from build123d import *


with BuildPart() as f1:
    # F0 (on Front) → F1 (revolve)
    with BuildSketch(Plane.XZ):
        with BuildLine():
            ThreePointArc((9, 2), (9.736068, 1.118034), (10, 0))
            Line((10, 0), (11, 0))
            Line((11, 0), (11, 3.25))
            ThreePointArc((11, 3.25), (10.926777, 3.426777), (10.75, 3.5))
            Line((10.75, 3.5), (9.606548, 3.5))
            ThreePointArc((9.606548, 3.5), (9.429771, 3.426777), (9.356548, 3.25))
            Line((9.356548, 3.25), (9.356548, 3))
            Line((9.356548, 3), (9, 3))
            Line((9, 3), (9, 2))
        make_face()
        with BuildLine():
            Line((11, 0), (10, 0))
            ThreePointArc((10, 0), (9.736068, -1.118034), (9, -2))
            Line((9, -2), (9, -3))
            Line((9, -3), (9.356548, -3))
            Line((9.356548, -3), (9.356548, -3.25))
            ThreePointArc((9.356548, -3.25), (9.429771, -3.426777), (9.606548, -3.5))
            Line((9.606548, -3.5), (10.75, -3.5))
            ThreePointArc((10.75, -3.5), (10.926777, -3.426777), (11, -3.25))
            Line((11, -3.25), (11, 0))
        make_face()
    revolve(axis=Axis((0, 0, -0.050428), (0, 0, -1)))


solid = f1.part
Part model, mm, in its own coordinate system. Coordinates: 2 decimals unless noted, no trailing zeros. Loops run counter-clockwise (first coordinate to the right, second up) from the corner with the lowest first, then second, coordinate; pieces in that order, holes last. Notation, with made-up numbers: (-21.75, -10) -> (-6.75, -10) arc R19 cw to (-6.75, 14) -> close; hole circle Ø9 at (65, 45). An arc over 180 degrees is marked (long way). Use a Markdown table: item, result. Add a question column.
Item 1: Pull direction Y, two halves, no side cores. Call faces 1 (the cylindrical face through (-1.172, -8.923, -2.507)), 2 (the cylindrical face through (-1.172, -8.923, 2.493)), 3 (the flat face through (-8, 6, 3.5)), 4 (the cylindrical face through (-2.38, 10.74, 0.05)): +Y half, -Y half, draft (parallel to the pull), parting line (faces both ways), or undercut.
Item 2: Flat gauge pins, fed straight in: P1, Ø4, axis at y = -3.5, z = -2.5, coming from the -X side; P2, Ø1, axis at y = -7.5, z = -0.5, coming from the -X side; P3, Ø2, axis at x = -6.5, z = -2, coming from the -Y side. Where does each tip first touch, or does it go through?
Item 3: Band-saw the part on A-A on z = 1.5. Write the cut outline in (x, y), plus the area to 3 significant figures.
Item 4: Probe probe 1 along Y at (x, z) = (0, -2.65); probe 2 along X at (y, z) = (0, -3.05). List the from-to ranges inside material, lowest first.
Geometry says:
| question | item | result |
|---|---|---|
| 1 | face 1 | undercut |
| 1 | face 2 | undercut |
| 1 | face 3 | draft |
| 1 | face 4 | parting line |
| 2 | P1 | x = -10.9 |
| 2 | P2 | x = -8.49 |
| 2 | P3 | y = -9.53 |
| 3 | outline | circle Ø22 at (0, 0); hole circle Ø19 at (0, 0) |
| 3 | area | 96.6 mm² |
| 4 | probe 1 | -11 to -9, 9 to 11 |
| 4 | probe 2 | -11 to -9.36, 9.36 to 11 |
